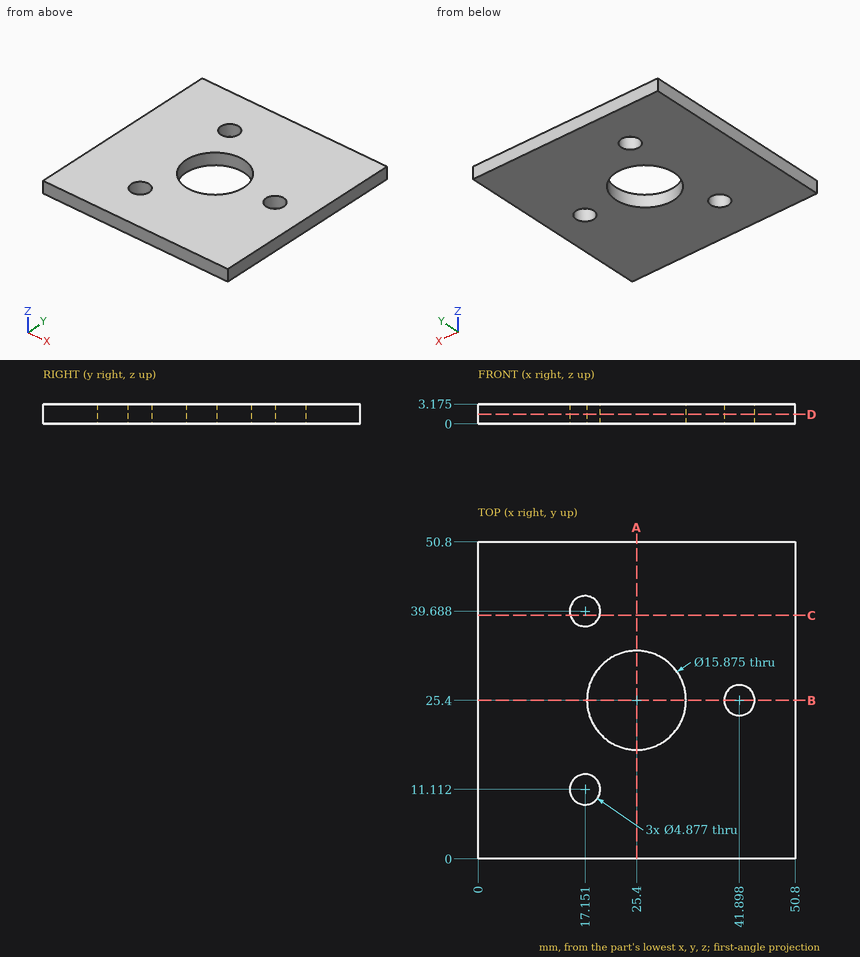
Input: dimensioned drawing with shaded views. Units: mm. Origin: part minimum x, y, z. Coordinates: 2 decimals unless noted, no trailing zeros. Loops run counter-clockwise (first coordinate to the right, second up) from the corner with the lowest first, then second, coordinate; pieces in that order, holes last. Notation, with made-up numbers: (-0.75, -19.75) -> (28.25, -19.75) arc R16 cw to (28.25, -3.75) -> close; hole circle Ø4 at (31.5, 48). An arc over 180 degrees is marked (long way). Use a Markdown table: item, result. Add a question column.
(1) Section query D-D, the plane z = 1.5. Return loops of the section in (x, y) (1 decimal).
(2) Section query C-C, the plane y = 39. Return loops of the section in (x, z) (1 decimal).
(3) Pin query (flat end, axial travel): pin 1 Ø4.5 at (x, y) = (41.9, 25.4) entering from -Z (3 decimals). Return the tip coordinate at first contact, or that it passes through.
(4) Section query A-A, the plane x = 25.4. Return loops of the section in (y, z) (1 decimal).
(5) Line query: line 1 along Y through (x, z) = (25.4, 1.45); line 2 along X through (y, z) = (24, 0.7) (1 decimal); line 3 along X through (y, z) = (9.5, 2.8). Output: solid intervals per line, ascending.
(6) Section query B-B, the plane y = 25.4. Return loops of the section in (x, z) (1 decimal).
Answer:
| question | item | result |
|---|---|---|
| 1 | outline | (0, 0) -> (50.8, 0) -> (50.8, 50.8) -> (0, 50.8) -> close; hole circle Ø4.9 at (17.2, 11.1); hole circle Ø4.9 at (17.2, 39.7); hole circle Ø15.9 at (25.4, 25.4); hole circle Ø4.9 at (41.9, 25.4) |
| 2 | outline | (0, 0) -> (14.8, 0) -> (14.8, 3.2) -> (0, 3.2) -> close; (19.5, 0) -> (50.8, 0) -> (50.8, 3.2) -> (19.5, 3.2) -> close |
| 3 | pin 1 | passes through |
| 4 | outline | (0, 0) -> (17.5, 0) -> (17.5, 3.2) -> (0, 3.2) -> close; (33.3, 0) -> (50.8, 0) -> (50.8, 3.2) -> (33.3, 3.2) -> close |
| 5 | line 1 | y = 0 to 17.46, 33.34 to 50.8 |
| 5 | line 2 | x = 0 to 17.6, 33.2 to 39.9, 43.9 to 50.8 |
| 5 | line 3 | x = 0 to 15.32, 18.98 to 50.8 |
| 6 | outline | (0, 0) -> (17.5, 0) -> (17.5, 3.2) -> (0, 3.2) -> close; (33.3, 0) -> (39.5, 0) -> (39.5, 3.2) -> (33.3, 3.2) -> close; (44.3, 0) -> (50.8, 0) -> (50.8, 3.2) -> (44.3, 3.2) -> close |
